```python
from build123d import *

# Parameters (mm, degrees)
SKETCH_1_W          = 50
SKETCH_1_H          = 42
EXTRUDE_1_DEPTH     = 2
SKETCH_2_W          = 50
SKETCH_2_H          = 110
EXTRUDE_2_DEPTH     = 2
CUT_EXTRUDE_1_REACH = 123.083
SKETCH_3_R          = 2.5
CUT_EXTRUDE_2_REACH = 123.083
SKETCH_4_R          = 13
FILLET_1_R          = 2
SKETCH_5_W          = 30
SKETCH_5_H          = 2
EXTRUDE_3_DEPTH     = 18
SKETCH_6_W          = 30
SKETCH_6_H          = 42
EXTRUDE_4_DEPTH     = 2
FILLET_2_R          = 2
CUT_EXTRUDE_3_REACH = 144.734
SKETCH_7_R          = 2.5
CUT_EXTRUDE_4_REACH = 128.732
SKETCH_8_R          = 2.5


with BuildPart() as part:
    # Sketch 1 → Extrude 1 (new body)
    with BuildSketch(Plane.XY):
        Rectangle(SKETCH_1_W, SKETCH_1_H)
        with BuildLine():
            Line((-17.5, 11), (-17.5, -11))
            ThreePointArc((-17.5, -11), (-15, -13.5), (-12.5, -11))
            Line((-12.5, -11), (-12.5, 11))
            ThreePointArc((-12.5, 11), (-15, 13.5), (-17.5, 11))
        make_face(mode=Mode.SUBTRACT)
        with BuildLine():
            Line((12.5, 13), (12.5, -13))
            ThreePointArc((12.5, -13), (15, -15.5), (17.5, -13))
            Line((17.5, -13), (17.5, 13))
            ThreePointArc((17.5, 13), (15, 15.5), (12.5, 13))
        make_face(mode=Mode.SUBTRACT)
    extrude(amount=EXTRUDE_1_DEPTH)

    # Sketch 2 → Extrude 2 (add)
    with BuildSketch(Plane.XZ.offset(21)):
        with Locations((0, 55)):
            Rectangle(SKETCH_2_W, SKETCH_2_H)
    extrude(amount=EXTRUDE_2_DEPTH)

    # Sketch 3 → Cut-Extrude 1 (cut, up to next)
    with BuildSketch(Plane.XZ.offset(23), mode=Mode.PRIVATE) as cut_extrude_1_sk1:
        with Locations(Location((17.76, 79.25, 0), (0, 0, 270))):
            Circle(SKETCH_3_R)
    cut_extrude_1_tool1 = extrude(cut_extrude_1_sk1.sketch, amount=-CUT_EXTRUDE_1_REACH, mode=Mode.PRIVATE) & part.part
    # Sketch 3 → Cut-Extrude 1 (cut, up to next)
    with BuildSketch(Plane.XZ.offset(23), mode=Mode.PRIVATE) as cut_extrude_1_sk2:
        with Locations(Location((-17.76, 79.25, 0), (0, 0, 270))):
            Circle(SKETCH_3_R)
    cut_extrude_1_tool2 = extrude(cut_extrude_1_sk2.sketch, amount=-CUT_EXTRUDE_1_REACH, mode=Mode.PRIVATE) & part.part
    # Sketch 3 → Cut-Extrude 1 (cut, up to next)
    with BuildSketch(Plane.XZ.offset(23), mode=Mode.PRIVATE) as cut_extrude_1_sk3:
        with Locations(Location((0, 61.49, 0), (0, 0, 270))):
            Circle(SKETCH_3_R)
    cut_extrude_1_tool3 = extrude(cut_extrude_1_sk3.sketch, amount=-CUT_EXTRUDE_1_REACH, mode=Mode.PRIVATE) & part.part
    # Sketch 3 → Cut-Extrude 1 (cut, up to next)
    with BuildSketch(Plane.XZ.offset(23), mode=Mode.PRIVATE) as cut_extrude_1_sk4:
        with Locations(Location((0, 97.01, 0), (0, 0, 270))):
            Circle(SKETCH_3_R)
    cut_extrude_1_tool4 = extrude(cut_extrude_1_sk4.sketch, amount=-CUT_EXTRUDE_1_REACH, mode=Mode.PRIVATE) & part.part
    add(cut_extrude_1_tool1.solids().sort_by_distance((17.76, -23, 79.25))[0], mode=Mode.SUBTRACT)
    add(cut_extrude_1_tool2.solids().sort_by_distance((-17.76, -23, 79.25))[0], mode=Mode.SUBTRACT)
    add(cut_extrude_1_tool3.solids().sort_by_distance((0, -23, 61.49))[0], mode=Mode.SUBTRACT)
    add(cut_extrude_1_tool4.solids().sort_by_distance((0, -23, 97.01))[0], mode=Mode.SUBTRACT)

    # Sketch 4 → Cut-Extrude 2 (cut, up to next)
    with BuildSketch(Plane.XZ.offset(23), mode=Mode.PRIVATE) as cut_extrude_2_sk1:
        with Locations(Location((0, 79.25, 0), (0, 0, 270))):
            Circle(SKETCH_4_R)
    cut_extrude_2_tool1 = extrude(cut_extrude_2_sk1.sketch, amount=-CUT_EXTRUDE_2_REACH, mode=Mode.PRIVATE) & part.part
    add(cut_extrude_2_tool1.solids().sort_by_distance((0, -23, 79.25))[0], mode=Mode.SUBTRACT)

    # Fillet 1
    fillet_1_edges = [part.edges().sort_by_distance(p)[0] for p in [
        (0, -23, 0),
    ]]
    fillet(fillet_1_edges, radius=FILLET_1_R)

    # Sketch 5 → Extrude 3 (add)
    with BuildSketch(Plane(origin=(25, 0, 0), x_dir=(0, 0, -1), z_dir=(1, 0, 0))):
        with Locations((-58.75, -22)):
            Rectangle(SKETCH_5_W, SKETCH_5_H)
    extrude_3 = extrude(amount=EXTRUDE_3_DEPTH)

    # Sketch 6 → Extrude 4 (add)
    with BuildSketch(Plane(origin=(43, 0, 0), x_dir=(0, 0, -1), z_dir=(1, 0, 0))):
        with Locations((-58.75, -2)):
            Rectangle(SKETCH_6_W, SKETCH_6_H)
    extrude_4 = extrude(amount=EXTRUDE_4_DEPTH)

    # Mirror 1: Extrude 3, Extrude 4 across plane
    add(extrude_3.mirror(Plane(origin=(0, 0, 0), x_dir=(0, 0, 1), z_dir=(1, 0, 0))))
    add(extrude_4.mirror(Plane(origin=(0, 0, 0), x_dir=(0, 0, 1), z_dir=(1, 0, 0))))

    # Fillet 2
    fillet_2_edges = [part.edges().sort_by_distance(p)[0] for p in [
        (45, -23, 58.75),
        (-45, -23, 58.75),
    ]]
    fillet(fillet_2_edges, radius=FILLET_2_R)

    # Sketch 7 → Cut-Extrude 3 (cut, up to next)
    with BuildSketch(Plane(origin=(-43, 0, 0), x_dir=(0, 0, -1), z_dir=(1, 0, 0)), mode=Mode.PRIVATE) as cut_extrude_3_sk1:
        with Locations((-48.75, 11.67)):
            Circle(SKETCH_7_R)
    cut_extrude_3_tool1 = extrude(cut_extrude_3_sk1.sketch, amount=-CUT_EXTRUDE_3_REACH, mode=Mode.PRIVATE) & part.part
    cut_extrude_3 = cut_extrude_3_tool1.solids().sort_by_distance((-43, 11.67, 48.75))[0]
    add(cut_extrude_3, mode=Mode.SUBTRACT)

    # Mirror 2: Cut-Extrude 3 across plane
    add(cut_extrude_3.mirror(Plane(origin=(0, 0, 0), x_dir=(0, 0, 1), z_dir=(1, 0, 0))), mode=Mode.SUBTRACT)

    # Sketch 8 → Cut-Extrude 4 (cut, up to next)
    with BuildSketch(Plane.XZ.offset(23), mode=Mode.PRIVATE) as cut_extrude_4_sk1:
        with Locations(Location((10, 12, 0), (0, 0, 270))):
            Circle(SKETCH_8_R)
    cut_extrude_4_tool1 = extrude(cut_extrude_4_sk1.sketch, amount=-CUT_EXTRUDE_4_REACH, mode=Mode.PRIVATE) & part.part
    # Sketch 8 → Cut-Extrude 4 (cut, up to next)
    with BuildSketch(Plane.XZ.offset(23), mode=Mode.PRIVATE) as cut_extrude_4_sk2:
        with Locations(Location((-10, 12, 0), (0, 0, 270))):
            Circle(SKETCH_8_R)
    cut_extrude_4_tool2 = extrude(cut_extrude_4_sk2.sketch, amount=-CUT_EXTRUDE_4_REACH, mode=Mode.PRIVATE) & part.part
    add(cut_extrude_4_tool1.solids().sort_by_distance((10, -23, 12))[0], mode=Mode.SUBTRACT)
    add(cut_extrude_4_tool2.solids().sort_by_distance((-10, -23, 12))[0], mode=Mode.SUBTRACT)


solid = part.part
```
CAD build for the part. Positions are in the model's coordinates, mm. A direction names the side the tool comes from. Round coordinates to 2 decimals unless told otherwise and drop trailing zeros. Loops run counter-clockwise (first coordinate to the right, second up) from the corner with the lowest first, then second, coordinate; pieces in that order, holes last. Notation, with made-up numbers: (-4, 1.5) - (43, 1.5) arc R21 ccw to (43, 18.5) - close; hole circle Ø5 at (-33, 1). An arc over 180 degrees is marked (long way). Return JSON: item names as keys, results as strings. Group by question number.
Q1. Band-saw the part on D-D on x = -10. Give the cut face in (y, z).
Q2. Flat gauge pins, fed straight in: pin 1 Ø2 at (y, z) = (1, 1) entering from +X; pin 2 Ø2 at (y, z) = (-15.5, 41) entering from +X; pin 3 Ø6 at (x, y) = (-15.5, 15) entering from +Z; pin 4 Ø3 at (x, z) = (-14, 49.5) entering from +Y. Where does each tip first touch, or does it go through?
Q3. Drill centre lines: line 1 along X through (y, z) = (-22.5, 79.25); line 2 along X through (y, z) = (-22.4, 12); line 3 along X through (y, z) = (-22.4, 97.01). Where is each one in solid material? Low to high. Write a range as [from, to].
Q4. Tool access for faces 1 (the face through (-25, -11, 1)), 2 (the face through (0, 0, 2)), 3 (the face through (-1, -21, 57)): list every direction of +Z, -Z, +X, -X, +Y, -Y with a clear straight run to the whole face (end or side of a thin tool).
Q5. Two-plate mould, pull along Z, no slides. Class faces 4 (the face through (-15.1, -13.5, 1)), 5 (the face through (-43.99, 10.71, 46.44)), 6 (the face through (-44, -7, 43.75)): +Z half, -Z half, draft (parallel to the pull), parting line (faces both ways), or undercut.
Q6. Band-saw the part on B-B on z = 12. Give the cut face in (x, y).
Q7. Band-saw the part on C-C on x = 0. Give the cut face in (y, z).
Q8. Band-saw the part on A-A on y = -1.5. Give the cut face in (x, z).
Solutions:
{
 "1": {"outline": "(-23, 2) arc R2 ccw to (-21, 0) - (21, 0) - (21, 2) - (-21, 2) - (-21, 9.5) - (-23, 9.5) - close; (-23, 14.5) - (-21, 14.5) - (-21, 70.94) - (-23, 70.94) - close; (-23, 87.56) - (-21, 87.56) - (-21, 110) - (-23, 110) - close"},
 "2": {"pin 1": "stops at x = 25", "pin 2": "passes through", "pin 3": "stops at z = 2", "pin 4": "stops at y = -21"},
 "3": {"line 1": "x = [-25, -20.26], [-15.26, -13], [13, 15.26], [20.26, 25]", "line 2": "x = [-25, -12.5], [-7.5, 7.5], [12.5, 25]", "line 3": "x = [-25, -2.5], [2.5, 25]"},
 "4": {"face 1": "-Z, -X, +Y, -Y", "face 2": "+Z, +X, -X, +Y", "face 3": "+Z, +Y"},
 "5": {"face 4": "draft", "face 5": "undercut", "face 6": "-Z half"},
 "6": {"outline": "(-25, -23) - (-12.5, -23) - (-12.5, -21) - (-25, -21) - close; (-7.5, -23) - (7.5, -23) - (7.5, -21) - (-7.5, -21) - close; (12.5, -23) - (25, -23) - (25, -21) - (12.5, -21) - close"},
 "7": {"outline": "(-23, 2) arc R2 ccw to (-21, 0) - (21, 0) - (21, 2) - (-21, 2) - (-21, 58.99) - (-23, 58.99) - close; (-23, 63.99) - (-21, 63.99) - (-21, 66.25) - (-23, 66.25) - close; (-23, 92.25) - (-21, 92.25) - (-21, 94.51) - (-23, 94.51) - close; (-23, 99.51) - (-21, 99.51) - (-21, 110) - (-23, 110) - close"},
 "8": {"outline": "(-45, 43.75) - (-43, 43.75) - (-43, 73.75) - (-45, 73.75) - close; (-25, 0) - (-17.5, 0) - (-17.5, 2) - (-25, 2) - close; (-12.5, 0) - (12.5, 0) - (12.5, 2) - (-12.5, 2) - close; (17.5, 0) - (25, 0) - (25, 2) - (17.5, 2) - close; (43, 43.75) - (45, 43.75) - (45, 73.75) - (43, 73.75) - close"}
}
